The model under review builds one solid part; all positions refer to its coordinate system, in mm. Face numbers are marked on the shaded views. A direction names the side the tool comes from. Give positions to 0.01 mm unless a question says otherwise; leave off trailing zeros. Loops run counter-clockwise (first coordinate to the right, second up) from the corner with the lowest first, then second, coordinate; pieces in that order, holes last. Notation, with made-up numbers: (1.5, 32) -> (19.5, 32) arc R15 ccw to (19.5, 58) -> close; hole circle Ø2 at (35.5, 52.25). An arc over 180 degrees is marked (long way). Write each question's results on one line, items separated by ' | '. Start each with the question number.
Q1. Insertion check: pin 1 Ø6.5 at (x, y) = (5.5, -87.5) entering from +Z; pin 2 Ø12 at (y, z) = (-17, -11.5) entering from -X; pin 3 Ø1.5 at (x, y) = (13.5, -38.5) entering from +Z. Each pin has a flat end and moves straight along its axis. Give the tip position at first contact, or say it passes through.
Q2. We need section B-B (z = -7.5). Give the number of separate pieces and of enclosed holes in the cut face, plus the area to 3 significant figures.
Q3. Wall thickness on L1, parallel to Y at x = -29.5, z = -12.75; L2, parallel to Y at x = -22, z = -7; L3, parallel to Z at x = -36.5, y = -128: over which ranges is each line inside the solid? List them lowest first. Write a range as [from, to].
Q4. Machinability: for the marked faces 1 and 2, which of the approach directions +Z, -Z, +X, -X, +Y, -Y give a long, thin tool a straight path to every point of the face, cutting with its end or side? Answer none if there is none.
Q5. We need section C-C (x = -6). Write out the cut boundary in (y, z).
Q6. We need section A-A (y = -105). Write out the cut boundary in (x, z), plus the area to 3 significant figures.
from build123d import *

# Parameters (mm, degrees)
F1_DEPTH = 140
F2_R     = 4
F3_DEPTH = 30
F4_R     = 4
F4_R_2   = 2
F5_DEPTH = 10


with BuildPart() as f1:
    # F0 (on Front) → F1 (new body)
    with BuildSketch(Plane.XZ):
        Polygon((2.0625628796, 5.9807691723), (0, 0), (-31.5625444055, 10.8848428354), (-45.9147356451, -17.5394751132), (29.6659134328, -17.5394751132), (10.4307364672, 5.9807691723), align=None)
    extrude(amount=F1_DEPTH)

    # F2 (on face) → F3 (cut)
    with BuildSketch(Plane(origin=(0, 0, 0), x_dir=(0.9453618412, 0, -0.3260229889), z_dir=(0.3260229889, 0, 0.9453618412))):
        with Locations((-23.3867340855, -10)):
            Circle(F2_R)
        with Locations((-28.3867340855, -50)):
            Circle(F2_R)
        with Locations((-23.3867340855, -130)):
            Circle(F2_R)
        with Locations((-18.3867340855, -90)):
            Circle(F2_R)
    extrude(amount=-F3_DEPTH, mode=Mode.SUBTRACT)

    # F4 (on face) → F5 (join)
    with BuildSketch(Plane(origin=(0, 0, 0), x_dir=(0.9453618412, 0, -0.3260229889), z_dir=(0.3260229889, 0, 0.9453618412))):
        with Locations((-23.3867340855, -10)):
            Circle(F4_R)
        with Locations((-23.3867340855, -10)):
            Circle(F4_R_2, mode=Mode.SUBTRACT)
        with Locations((-23.3867340855, -130)):
            Circle(F4_R)
        with Locations((-23.3867340855, -130)):
            Circle(F4_R_2, mode=Mode.SUBTRACT)
        with Locations((-28.3867340855, -50)):
            Circle(F4_R)
        with Locations((-28.3867340855, -50)):
            Circle(F4_R_2, mode=Mode.SUBTRACT)
        with Locations((-18.3867340855, -90)):
            Circle(F4_R)
        with Locations((-18.3867340855, -90)):
            Circle(F4_R_2, mode=Mode.SUBTRACT)
    extrude(amount=-F5_DEPTH)


solid = f1.part
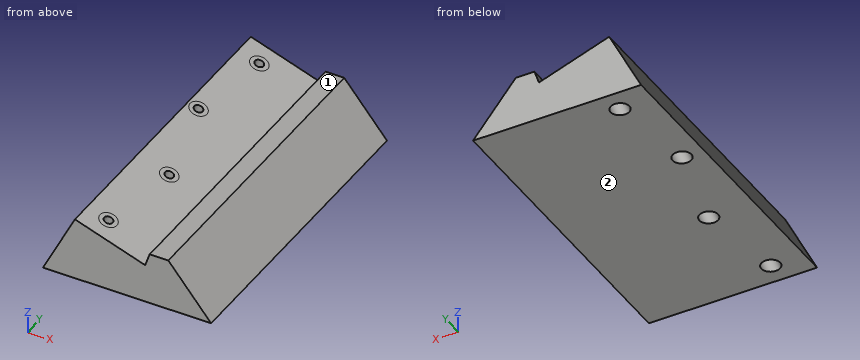
Output:
1) pin 1: z = 5.98 | pin 2: x = -45.89 | pin 3: z = 3.14
2) separate pieces: 1 | enclosed holes: 4 | area: 8,510 mm2
3) L1: [-140, -133.99], [-126.01, -13.99], [-6.01, 0] | L2: [-140, -94], [-86, 0] | L3: [-17.54, 1.11]
4) face 1: +Z, +X, +Y, -Y | face 2: -Z, +X, -X, +Y, -Y
5) outline: (-140, -17.54) -> (0, -17.54) -> (0, 2.07) -> (-140, 2.07) -> close
6) outline: (-45.91, -17.54) -> (29.67, -17.54) -> (10.43, 5.98) -> (2.06, 5.98) -> (0, 0) -> (-31.56, 10.88) -> close | area: 1,390 mm2
